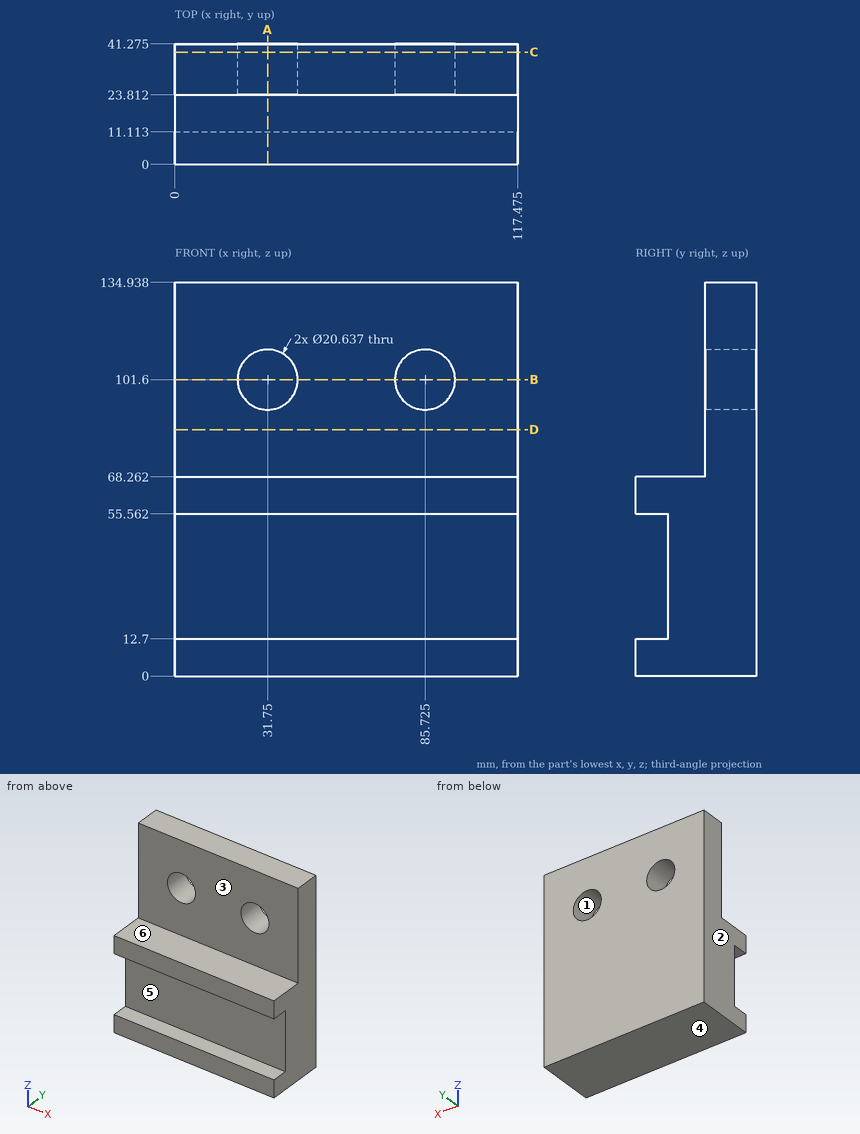
Answer from the drawing. Dimensions are ordinates in mm from the lowest x, y and z of the part. A direction names the side the tool comes from. Give positions to 0.01 mm unless a question says otherwise; leave off trailing zeros. Loops run counter-clockwise (first coordinate to the right, second up) from the corner with the lowest first, then second, coordinate; pieces in that order, holes last. Notation, with made-up numbers: (10, -20) -> (53, -20) arc R12 ccw to (53, -10) -> close; hole circle Ø10 at (-28.5, 66). An arc over 180 degrees is marked (long way). One line per question, with ' | ' between items. Start each with the question number.
1) Section D-D, the plane z = 84.5 is taken. Determine the outline of the cut face in (x, y) (1 decimal).
2) Section A-A, the plane x = 31.75 is taken. Determine the outline of the cut face in (y, z) (1 decimal).
3) Each of these flat-tipped pins is pushed along its axis until it touches: pin 1 (9 mm diameter, centred on x = 68, y = 6, fed in from +Z); pin 2 (6 mm diameter, centred on x = 89, z = 75, fed in from -Y); pin 3 (13 mm diameter, centred on x = 84, z = 42.5, fed in from -Y). Where does it stop, or does it pass through?
4) Determine the mould class of the marked faces 1, 2 and 3 for opening direction X: +X half, -X half, draft (parallel to the pull), parting line (faces both ways), or undercut.
5) Section B-B, the plane z = 101.6 is taken. Determine the outline of the cut face in (x, y) (1 decimal), then the cut area to 3 significant figures.
6) Section C-C, the plane y = 38.5 is taken. State how many separate pieces and enclosed holes the cut face has, then the cut area to 3 significant figures.
7) Straight lines are drawn through the part: L1, parallel to X at y = 30, z = 101 (1 decimal); L2, parallel to Z at x = 31, y = 27; L3, parallel to Z at x = 42, y = 2. For each, find the intervals that lie inside material, in ascending order.
8) For the marked faces 4, 5 and 6, determine the directions among +Z, -Z, +X, -X, +Y, -Y from which every point of the face is accessible in a straight line to the end or side of a thin tool.
Resolved:
1) outline: (0, 23.8) -> (117.5, 23.8) -> (117.5, 41.3) -> (0, 41.3) -> close
2) outline: (0, 0) -> (41.3, 0) -> (41.3, 91.3) -> (23.8, 91.3) -> (23.8, 68.3) -> (0, 68.3) -> (0, 55.6) -> (11.1, 55.6) -> (11.1, 12.7) -> (0, 12.7) -> close; (23.8, 111.9) -> (41.3, 111.9) -> (41.3, 134.9) -> (23.8, 134.9) -> close
3) pin 1: z = 68.26 | pin 2: y = 23.81 | pin 3: y = 11.11
4) face 1: undercut | face 2: -X half | face 3: draft
5) outline: (0, 23.8) -> (21.4, 23.8) -> (21.4, 41.3) -> (0, 41.3) -> close; (42.1, 23.8) -> (75.4, 23.8) -> (75.4, 41.3) -> (42.1, 41.3) -> close; (96, 23.8) -> (117.5, 23.8) -> (117.5, 41.3) -> (96, 41.3) -> close | area: 1,330 mm2
6) separate pieces: 1 | enclosed holes: 2 | area: 15,200 mm2
7) L1: 0 to 21.4, 42.1 to 75.4, 96 to 117.5 | L2: 0 to 91.31, 111.89 to 134.94 | L3: 0 to 12.7, 55.56 to 68.26
8) face 4: -Z, +X, -X, +Y, -Y | face 5: +X, -X, -Y | face 6: +Z, +X, -X, -Y
